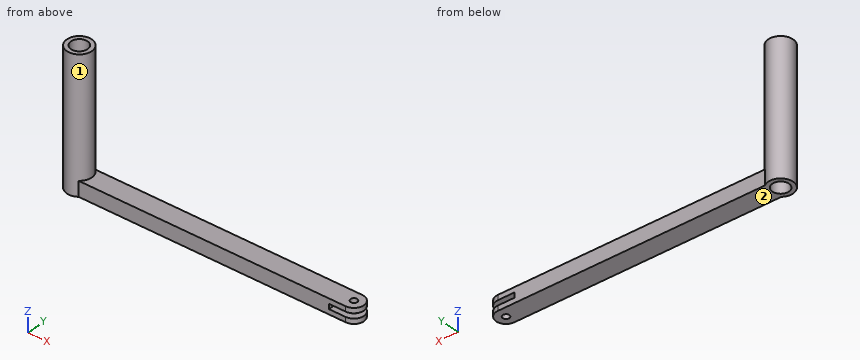
```python
from build123d import *

# Parameters (mm, degrees)
SKETCH_1_R          = 7.5
SKETCH_1_R_2        = 5
EXTRUDE_1_DEPTH     = 80
EXTRUDE_START       = -9
SKETCH_2_R          = 2
EXTRUDE_2_DEPTH     = 9
SKETCH_4_W          = 20
SKETCH_4_H          = 3
CUT_EXTRUDE_1_DEPTH = 20


with BuildPart() as part:
    # 草图1 → 凸台-拉伸1 (new body)
    with BuildSketch(Plane.XY):
        Circle(SKETCH_1_R)
        Circle(SKETCH_1_R_2, mode=Mode.SUBTRACT)
    extrude(amount=EXTRUDE_1_DEPTH)

    # 草图2 → 凸台-拉伸2 (add)
    with BuildSketch(Plane.XY.offset(9).offset(EXTRUDE_START)):
        with BuildLine():
            Line((164.5, -6), (4.5, -6))
            ThreePointArc((4.5, -6), (7.5, 0), (4.5, 6))
            Line((4.5, 6), (164.5, 6))
            ThreePointArc((164.5, 6), (170.5, 0), (164.5, -6))
        make_face()
        with Locations((164.5, 0)):
            Circle(SKETCH_2_R, mode=Mode.SUBTRACT)
    extrude(amount=EXTRUDE_2_DEPTH)

    # 草图4 → 切除-拉伸1 (cut)
    with BuildSketch(Plane(origin=(0, 6, 0), x_dir=(1, 0, 0), z_dir=(0, 1, 0))):
        with Locations((164.5, -4.5)):
            Rectangle(SKETCH_4_W, SKETCH_4_H)
    extrude(amount=-CUT_EXTRUDE_1_DEPTH, mode=Mode.SUBTRACT)


solid = part.part
```
Input: part model. Units: mm. Frame: model coordinates. Face numbers are marked on the shaded views. A direction names the side the tool comes from. Round coordinates to 2 decimals unless told otherwise and drop trailing zeros. Write each loop counter-clockwise with the first axis right and the second up, starting at its lowest first coordinate (ties: lowest second). Pieces come first, ordered by that corner, then holes. Notation, with made-up numbers: M 63,16.25 L 88,16.25 A37 cw 88,52.25 Z; hole C 18,-1 d7. An arc over 180 degrees is marked long. Write each question's results on one line, items separated by ' | '.
Q1. Section query C-C (z = 14.5). Return loops of the section in (x, y), and give its area (3 significant figures).
Results:
outline: C 0,0 d15; hole C 0,0 d10 | area: 98.2 mm^2
Q2. Section query B-B (x = 0). Return loops of the section in (y, z).
Results:
outline: M -7.5,0 L -5,0 L -5,80 L -7.5,80 Z; M 5,0 L 7.5,0 L 7.5,80 L 5,80 Z
Q3. Pin query (flat end, axial travel): P1, Ø5, axis at y = -5.5, z = 60, coming from the +X side; P2, Ø8, axis at y = 1, z = 37, coming from the -X side; P3, Ø2, axis at x = 20.5, y = -4.5, coming from the +Z side; P4, Ø3, axis at y = 5, z = 31.5, coming from the +X side. Return the tip coordinate at first contact, or that it passes through.
Results:
P1: stops at x = 6.87 | P2: stops at x = -7.5 | P3: stops at z = 9 | P4: stops at x = 6.63
Q4. Section query D-D (x = 22.5). Return loops of the section in (y, z).
Results:
outline: M -6,0 L 6,0 L 6,9 L -6,9 Z
Q5. Line query: line 1 along Y through (x, z) = (164.5, 7.55); line 2 along Y through (x, z) = (0, 26); line 3 along X through (y, z) = (1.75, 7.5). Output: solid intervals per line, ascending.
Results:
line 1: y = -6 to -2, 2 to 6 | line 2: y = -7.5 to -5, 5 to 7.5 | line 3: x = -7.29 to -4.68, 4.68 to 163.53, 165.47 to 170.24
Q6. Section query A-A (y = 0). Return loops of the section in (x, z).
Results:
outline: M -7.5,0 L -5,0 L -5,80 L -7.5,80 Z; M 5,0 L 162.5,0 L 162.5,3 L 154.5,3 L 154.5,6 L 162.5,6 L 162.5,9 L 7.5,9 L 7.5,80 L 5,80 Z; M 166.5,0 L 170.5,0 L 170.5,3 L 166.5,3 Z; M 166.5,6 L 170.5,6 L 170.5,9 L 166.5,9 Z
Q7. Access query for the marked faces 1 and 2. Directions: +Z, -Z, +X, -X, +Y, -Y. A direction counts if a zero-diameter tool reaches every point of the face in a straight line with its end or side. Return the directions, or none.
Results:
face 1: +Z | face 2: -Z, +X, -X, +Y, -Y
